Could you check a few things on this model? Use its own coordinates, in mm. Face numbers are marked on the shaded views. A direction names the side the tool comes from. Give positions to 0.01 mm unless a question says otherwise; leave off trailing zeros. Loops run counter-clockwise (first coordinate to the right, second up) from the corner with the lowest first, then second, coordinate; pieces in that order, holes last. Notation, with made-up numbers: M 6,52 L 60,52 A23 ccw 60,78 Z; hole C 42,-35.75 d8. An arc over 180 degrees is marked long. Use a Markdown table: item, result. Add a question column.
1) Suppose I cut it at D-D on x = -365. List the corners of the cut face in (y, z) for me.
2) Which directions (+Z, -Z, +X, -X, +Y, -Y) give clear straight access to the entire face, cutting with the end or side of a thin tool? Please do the marked faces 4 and 5.
3) Suppose I cut it at C-C on z = 441.5. List the corners of the cut face in (x, y) for me.
4) We'd pull the mould along Y, two halves only. Please class the marked faces 1, 2 and 3: +Y half, -Y half, draft (parallel to the pull), parting line (faces both ways), or undercut.
5) Suppose I cut it at A-A on z = 115.5. List the corners of the cut face in (x, y) for me.
6) Will these pins go through, and if not, where does the flat tip stop? pin 1 Ø12 at (x, y) = (-439.5, 874) entering from +Z; pin 2 Ø0.8 at (x, y) = (-499.5, 816) entering from -Z; pin 3 Ø6.5 at (x, z) = (-133, 687.5) entering from -Y.
7) If I drill on line 1 along Z through (x, y) = (-197, 156); line 2 along Z through (x, y) = (-436, 534.5); line 3 along X through (y, z) = (714, 921), over which ranges is the centre line in solid material (lowest first)? Write a range as [from, to].
8) Suppose I cut it at B-B on y = 170.5. List the corners of the cut face in (x, z) for me.
```python
from build123d import *

# Parameters (mm, degrees)
F0_W      = 500
F0_H      = 1000
F1_DEPTH  = 1900
F2_W      = 900
F2_H      = 350
F3_DEPTH  = 500
F4_W      = 400
F4_H      = 350
F5_DEPTH  = 1000
F6_W      = 405.736053
F6_H      = 230
F7_DEPTH  = 500
F8_DEPTH  = 500
F9_W      = 428.243608
F9_H      = 413.254976
F10_DEPTH = 200
F11_W     = 85.769325
F11_H     = 401.872158
F12_DEPTH = 500
F13_W     = 400
F13_H     = 230
F14_DEPTH = 50
F15_DEPTH = 85


with BuildPart() as f1:
    # F0 (on Top) → F1 (new body)
    with BuildSketch(Plane.XY):
        with Locations((-250, 500)):
            Rectangle(F0_W, F0_H)
    extrude(amount=F1_DEPTH)

    # F2 (on face) → F3 (cut)
    with BuildSketch(Plane.YZ):
        with Locations((500, 175)):
            Rectangle(F2_W, F2_H)
    extrude(amount=-F3_DEPTH, mode=Mode.SUBTRACT)

    # F4 (on face) → F5 (cut)
    with BuildSketch(Plane.XZ):
        with Locations((-250, 175)):
            Rectangle(F4_W, F4_H)
    extrude(amount=-F5_DEPTH, mode=Mode.SUBTRACT)

    # F6 (on face) → F7 (cut)
    with BuildSketch(Plane.YZ):
        with Locations((252.868026, 515)):
            Rectangle(F6_W, F6_H)
    extrude(amount=-F7_DEPTH, mode=Mode.SUBTRACT)

    # F6 (on face) → F8 (cut)
    with BuildSketch(Plane.YZ):
        with BuildLine():
            Line((500, 1657.026792), (500, 1900))
            Line((500, 1900), (0, 1900))
            Line((0, 1900), (0, 680))
            Line((0, 680), (50, 680))
            Line((50, 680), (455.736053, 680))
            Line((455.736053, 680), (505.736053, 680))
            Line((505.736053, 680), (505.736053, 692.793548))
            Line((505.736053, 692.793548), (544.31802, 722.311735))
            Line((544.31802, 722.311735), (544.31802, 876.871645))
            Line((544.31802, 876.871645), (505.736053, 905.245364))
            ThreePointArc((505.736053, 905.245364), (564.785088, 1077.27253), (703.88782, 1194.450021))
            Line((703.88782, 1194.450021), (792.619646, 1488.100433))
            Line((792.619646, 1488.100433), (500, 1657.026792))
        make_face()
    extrude(amount=-F8_DEPTH, mode=Mode.SUBTRACT)

    # F9 (on face) → F10 (cut)
    with BuildSketch(Plane.XY.offset(1900)):
        with Locations((-253.211826, 750)):
            Rectangle(F9_W, F9_H)
    extrude(amount=-F10_DEPTH, mode=Mode.SUBTRACT)

    # F11 (on face) → F12 (cut)
    with BuildSketch(Plane(origin=(0, 1000, 0), x_dir=(-1, 0, 0), z_dir=(0, 1, 0))):
        with Locations((457.115338, 893.803358)):
            Rectangle(F11_W, F11_H)
    extrude(amount=-F12_DEPTH, mode=Mode.SUBTRACT)

    # F13 (on face) → F14 (cut)
    with BuildSketch(Plane.XZ):
        with Locations((-250, 515)):
            Rectangle(F13_W, F13_H)
    extrude(amount=-F14_DEPTH, mode=Mode.SUBTRACT)

    # F12_face (on face) → F15 (join)
    with BuildSketch(Plane(origin=(-414.230675, 767.243571, 893.578105), x_dir=(0, -1, 0), z_dir=(-1, 0, 0))):
        with BuildLine():
            Line((-232.756429, 201.161332), (-232.756429, -200.710826))
            Line((-232.756429, -200.710826), (261.411147, -200.710826))
            Line((261.411147, -200.710826), (222.925551, -171.26637))
            Line((222.925551, -171.26637), (222.925551, -16.70646))
            Line((222.925551, -16.70646), (261.507518, 11.667259))
            ThreePointArc((261.507518, 11.667259), (239.989786, 111.877202), (189.656997, 201.161332))
            Line((189.656997, 201.161332), (-232.756429, 201.161332))
        make_face()
    extrude(amount=F15_DEPTH)


solid = f1.part
```
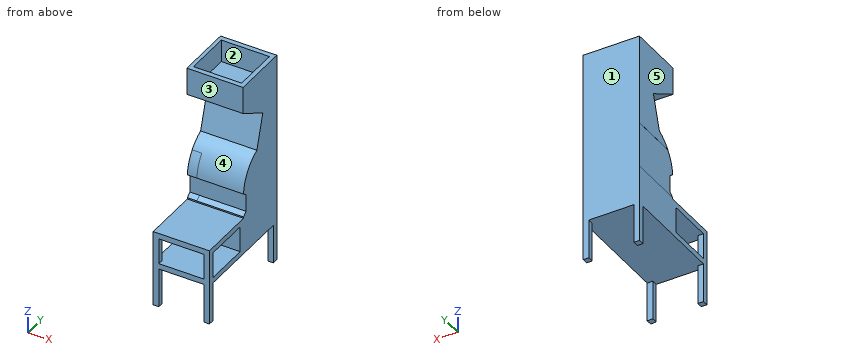
Answer block:
| question | item | result |
|---|---|---|
| 1 | outline | M 0,350 L 1000,350 L 1000,1900 L 956.63,1900 L 956.63,1700 L 543.37,1700 L 543.37,1900 L 500,1900 L 500,1657.03 L 792.62,1488.1 L 703.89,1194.45 A340.89 ccw 505.74,905.25 L 544.32,876.87 L 544.32,722.31 L 505.74,692.79 L 505.74,680 L 0,680 L 0,630 L 455.74,630 L 455.74,400 L 0,400 Z |
| 2 | face 4 | +X, -X, -Y |
| 2 | face 5 | +Z, -Z, -X, +Y, -Y |
| 3 | outline | M -500,0 L -450,0 L -450,50 L -500,50 Z; M -500,455.74 L 0,455.74 L 0,1000 L -500,1000 Z; M -50,0 L 0,0 L 0,50 L -50,50 Z |
| 4 | face 1 | +Y half |
| 4 | face 2 | undercut |
| 4 | face 3 | -Y half |
| 5 | outline | M -500,0 L -450,0 L -450,50 L -500,50 Z; M -500,950 L -450,950 L -450,1000 L -500,1000 Z; M -50,0 L 0,0 L 0,50 L -50,50 Z; M -50,950 L 0,950 L 0,1000 L -50,1000 Z |
| 6 | pin 1 | stops at z = 1700 |
| 6 | pin 2 | stops at z = 350 |
| 6 | pin 3 | stops at y = 505.74 |
| 7 | line 1 | z = [350, 400], [630, 680] |
| 7 | line 2 | z = [350, 714.8], [884.09, 1023.07], [1637.11, 1900] |
| 7 | line 3 | x = [-499.23, 0] |
| 8 | outline | M -500,350 L 0,350 L 0,400 L -500,400 Z; M -500,630 L 0,630 L 0,680 L -500,680 Z |
